```python
from build123d import *

# Parameters (mm, degrees)
SKETCH1_W           = 192
SKETCH1_H           = 42
SKETCH1_R           = 1.6
SKETCH1_R_2         = 11.5
BOSS_EXTRUDE1_DEPTH = 2


with BuildPart() as part:
    # Sketch1 → Boss-Extrude1 (new body)
    with BuildSketch(Plane(origin=(0, 0, 0), x_dir=(1, 0, 0), z_dir=(0, 1, 0))):
        Rectangle(SKETCH1_W, SKETCH1_H)
        with Locations(Location((-90.5, -15.5, 0), (0, 0, 270))):
            Circle(SKETCH1_R, mode=Mode.SUBTRACT)
        with Locations(Location((-59.5, -15.5, 0), (0, 0, 270))):
            Circle(SKETCH1_R, mode=Mode.SUBTRACT)
        with Locations(Location((59.5, -15.5, 0), (0, 0, 270))):
            Circle(SKETCH1_R, mode=Mode.SUBTRACT)
        with Locations(Location((90.5, -15.5, 0), (0, 0, 270))):
            Circle(SKETCH1_R, mode=Mode.SUBTRACT)
        with Locations(Location((-75, 0, 0), (0, 0, 270))):
            Circle(SKETCH1_R_2, mode=Mode.SUBTRACT)
        with Locations(Location((-90.5, 15.5, 0), (0, 0, 270))):
            Circle(SKETCH1_R, mode=Mode.SUBTRACT)
        with Locations(Location((-59.5, 15.5, 0), (0, 0, 270))):
            Circle(SKETCH1_R, mode=Mode.SUBTRACT)
        with Locations(Location((75, 0, 0), (0, 0, 270))):
            Circle(SKETCH1_R_2, mode=Mode.SUBTRACT)
        with Locations(Location((59.5, 15.5, 0), (0, 0, 270))):
            Circle(SKETCH1_R, mode=Mode.SUBTRACT)
        with Locations(Location((90.5, 15.5, 0), (0, 0, 270))):
            Circle(SKETCH1_R, mode=Mode.SUBTRACT)
    extrude(amount=BOSS_EXTRUDE1_DEPTH)


solid = part.part
```
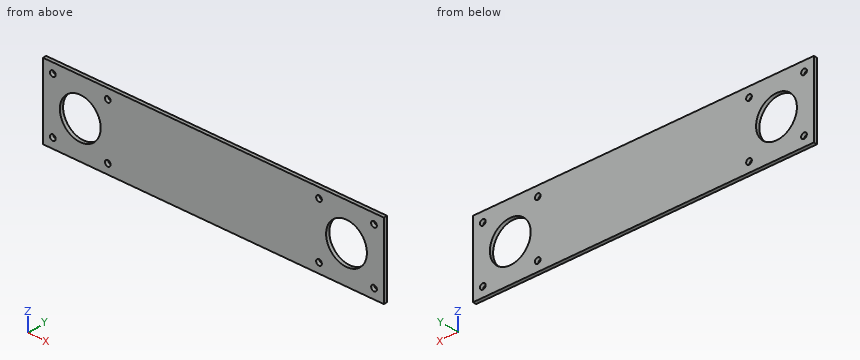
Work out the finished part from the listing and answer in its coordinate system (mm). Give positions to 0.01 mm unless a question says otherwise; leave off trailing zeros. Write each loop counter-clockwise with the first axis right and the second up, starting at its lowest first coordinate (ties: lowest second). Pieces come first, ordered by that corner, then holes. Notation, with made-up numbers: (74, 36.25) -> (110, 36.25) arc R29 ccw to (110, 57.25) -> close; hole circle Ø3 at (57.25, 27.25). An arc over 180 degrees is marked (long way). Write each question's results on one line, items separated by ' | '.
1. Find section D-D on y = 1.6. Give the number of separate pieces and of enclosed holes in the cut face, and give its area (3 significant figures).
Data:
separate pieces: 1 | enclosed holes: 10 | area: 7,170 mm^2
2. Find section B-B on z = 15.5. Determine the outline of the cut face in (x, y).
Data:
outline: (-96, 0) -> (-92.1, 0) -> (-92.1, 2) -> (-96, 2) -> close; (-88.9, 0) -> (-61.1, 0) -> (-61.1, 2) -> (-88.9, 2) -> close; (-57.9, 0) -> (57.9, 0) -> (57.9, 2) -> (-57.9, 2) -> close; (61.1, 0) -> (88.9, 0) -> (88.9, 2) -> (61.1, 2) -> close; (92.1, 0) -> (96, 0) -> (96, 2) -> (92.1, 2) -> close
3. Find section C-C on x = -75. Determine the outline of the cut face in (y, z), and give its area (3 significant figures).
Data:
outline: (0, -21) -> (2, -21) -> (2, -11.5) -> (0, -11.5) -> close; (0, 11.5) -> (2, 11.5) -> (2, 21) -> (0, 21) -> close | area: 38.0 mm^2
4. Find section A-A on x = 59.5. Determine the outline of the cut face in (y, z).
Data:
outline: (0, -21) -> (2, -21) -> (2, -17.1) -> (0, -17.1) -> close; (0, -13.9) -> (2, -13.9) -> (2, 13.9) -> (0, 13.9) -> close; (0, 17.1) -> (2, 17.1) -> (2, 21) -> (0, 21) -> close
5. Straight lines are drawn through the part: L1, parallel to X at y = 0.4, z = -15.5; L2, parallel to Z at x = 90.5, y = 0.5; L3, parallel to X at y = 1.6, z = 0. For each, find the intervals that lie inside material, in ascending order.
Data:
L1: -96 to -92.1, -88.9 to -61.1, -57.9 to 57.9, 61.1 to 88.9, 92.1 to 96 | L2: -21 to -17.1, -13.9 to 13.9, 17.1 to 21 | L3: -96 to -86.5, -63.5 to 63.5, 86.5 to 96
